```python
from build123d import *

# Parameters (mm, degrees)
BOSS_EXTRUDE1_DEPTH = 2
BOSS_EXTRUDE2_DEPTH = 8
BOSS_EXTRUDE3_DEPTH = 2.5
CHAMFER1_SIZE       = 2.5
SKETCH5_R           = 1.75
CUT_EXTRUDE1_DEPTH  = 123.114698641


with BuildPart() as part:
    # Sketch1 → Boss-Extrude1 (new body)
    with BuildSketch(Plane.XY):
        with BuildLine():
            Line((-43, -35.867648288), (-43, 1))
            Line((-43, 1), (-114.701591379, 1))
            ThreePointArc((-114.701591379, 1), (-116.115804942, 0.414213562), (-116.701591379, -1))
            Line((-116.701591379, -1), (-116.701591379, -4.677699552))
            Line((-116.701591379, -4.677699552), (-116.701591379, -27.177699552))
            ThreePointArc((-116.701591379, -27.177699552), (-116.179955267, -28.524711139), (-114.887151163, -29.169072838))
            Line((-114.887151163, -29.169072838), (-43, -35.867648288))
        make_face()
    extrude(amount=BOSS_EXTRUDE1_DEPTH)

    # Sketch3 → Boss-Extrude2 (add, symmetric)
    with BuildSketch(Plane(origin=(0, -17.899660586, 0), x_dir=(-1, 0, 0), z_dir=(0, -1, 0))):
        Polygon((42, -1), (42, 0), (43, 0), (43, -2), align=None)
    extrude(amount=BOSS_EXTRUDE2_DEPTH, both=True)

    # Sketch4 → Boss-Extrude3 (add)
    with BuildSketch(Plane(origin=(0, 0, 0), x_dir=(-1, 0, 0), z_dir=(0, 0, -1))):
        with BuildLine():
            Line((114.100916052, -24.89988692), (114.100916052, -10.60011308))
            ThreePointArc((114.100916052, -10.60011308), (113.605361745, -9.320452072), (112.377197846, -8.708308458))
            Line((112.377197846, -8.708308458), (43, -2.243615022))
            Line((43, -2.243615022), (43, -4.754445128))
            Line((43, -4.754445128), (111.600916052, -11.146803215))
            Line((111.600916052, -11.146803215), (111.600916052, -24.353196785))
            Line((111.600916052, -24.353196785), (43, -30.745554872))
            Line((43, -30.745554872), (43, -33.256384978))
            Line((43, -33.256384978), (112.377197846, -26.791691542))
            ThreePointArc((112.377197846, -26.791691542), (113.605361745, -26.179547928), (114.100916052, -24.89988692))
        make_face()
    extrude(amount=BOSS_EXTRUDE3_DEPTH)

    # Chamfer1
    chamfer1_edges = [part.edges().sort_by_distance(p)[0] for p in [
        (-77.300458026, -27.549375828, 0),
        (-111.600916052, -17.75, 0),
        (-77.300458026, -7.950624172, 0),
    ]]
    chamfer(chamfer1_edges, length=CHAMFER1_SIZE - 0.0001)  # a hair under: the kernel refuses the full size

    # Sketch5 → Cut-Extrude1 (cut, through all)
    with BuildSketch(Plane(origin=(0, 0, 0), x_dir=(-1, 0, 0), z_dir=(0, 0, -1))):
        with Locations((112.701591379, -3)):
            Circle(SKETCH5_R)
    extrude(amount=-CUT_EXTRUDE1_DEPTH, mode=Mode.SUBTRACT)


solid = part.part
```
Here's how the part is built. I have some questions about the finished solid (model axes, mm). A direction names the side the tool comes from. Coordinates: 2 decimals unless noted, no trailing zeros. Write each loop counter-clockwise with the first axis right and the second up, starting at its lowest first coordinate (ties: lowest second). Pieces come first, ordered by that corner, then holes. Notation, with made-up numbers: (52, 15.5) -> (61, 15.5) arc R34 cw to (61, 50.5) -> close; hole circle Ø11 at (-27.5, -13.5). An arc over 180 degrees is marked (long way). Use a Markdown table: item, result. Add a question column.
(1) Please list where these lines run through material, in increasing order: line 1 (Z direction, x = -101.5, y = -4); line 2 (Y direction, x = -101.5, z = -1.9); line 3 (Y direction, x = -65, z = -2).
(2) If we section it at C-C, the plane z = -1.4: Write out the boundary of the cut face in (x, y).
(3) For faces 1 (the flat face through (-88, -6, 0)), 2 (the flat face through (-77.67, -26.28, -1.27)), 3 (the flat face through (-80, -17, 2)), 4 (the flat face through (-116.702, -14, 1)), 5 (the cylindrical face through (-113.619, -9.335, -1.232)), which set-ups out of +Z, -Z, +X, -X, +Y, -Y let a thin tool reach every point of the face, with its end or its side?
(4) If we section it at A-A, the plane y = -3: Write out the boundary of the cut face in (x, z), and give its area (3 significant figures).
(5) I'm going to push flat-ended pins straight in: P1, Ø1, axis at x = -74, z = 0, coming from the -Y side; P2, Ø3, axis at x = -112.7, y = -3, coming from the +Z side; P3, Ø0.8, axis at x = -42.5, z = 0.5, coming from the +Y side; P4, Ø0.8, axis at y = -16.5, z = -1.5, coming from the -X side. Where does each tip first touch, or does it pass through?
(6) We'd pull the mould along Y, two halves only. Please class faces 6 (the flat face through (-43, -31, 0)), 7 (the flat face through (-110.4, -17.7, -1.3)), 8 (the cylindrical face through (-113.592, -26.194, -1.232)): +Y half, -Y half, draft (parallel to the pull), parting line (faces both ways), or undercut.
Outcome:
| question | item | result |
|---|---|---|
| 1 | line 1 | z = 0 to 2 |
| 1 | line 2 | y = -27.81 to -24.69, -10.81 to -7.69 |
| 1 | line 3 | y = -31.21 to -28.19, -7.31 to -4.29 |
| 2 | outline | (-114.1, -24.9) arc R1.9 ccw to (-112.38, -26.79) -> (-43, -33.26) -> (-43, -29.64) -> (-110.5, -23.35) -> (-110.5, -12.15) -> (-43, -5.86) -> (-43, -2.24) -> (-112.38, -8.71) arc R1.9 ccw to (-114.1, -10.6) -> close |
| 3 | face 1 | -Z, -X |
| 3 | face 2 | -Z, +X |
| 3 | face 3 | +Z, +X, -X, +Y, -Y |
| 3 | face 4 | +Z, -Z, -X, +Y, -Y |
| 3 | face 5 | -Z, -X, +Y |
| 4 | outline | (-116.7, 0) -> (-114.45, 0) -> (-114.45, 2) -> (-116.7, 2) -> close; (-110.95, 0) -> (-51.12, 0) -> (-51.12, -2.5) -> (-43, -2.5) -> (-43, 2) -> (-110.95, 2) -> close |
| 4 | area | 161 mm^2 |
| 5 | P1 | stops at y = -33.03 |
| 5 | P2 | passes through |
| 5 | P3 | stops at y = -9.9 |
| 5 | P4 | stops at x = -114.1 |
| 6 | face 6 | draft |
| 6 | face 7 | undercut |
| 6 | face 8 | -Y half |
